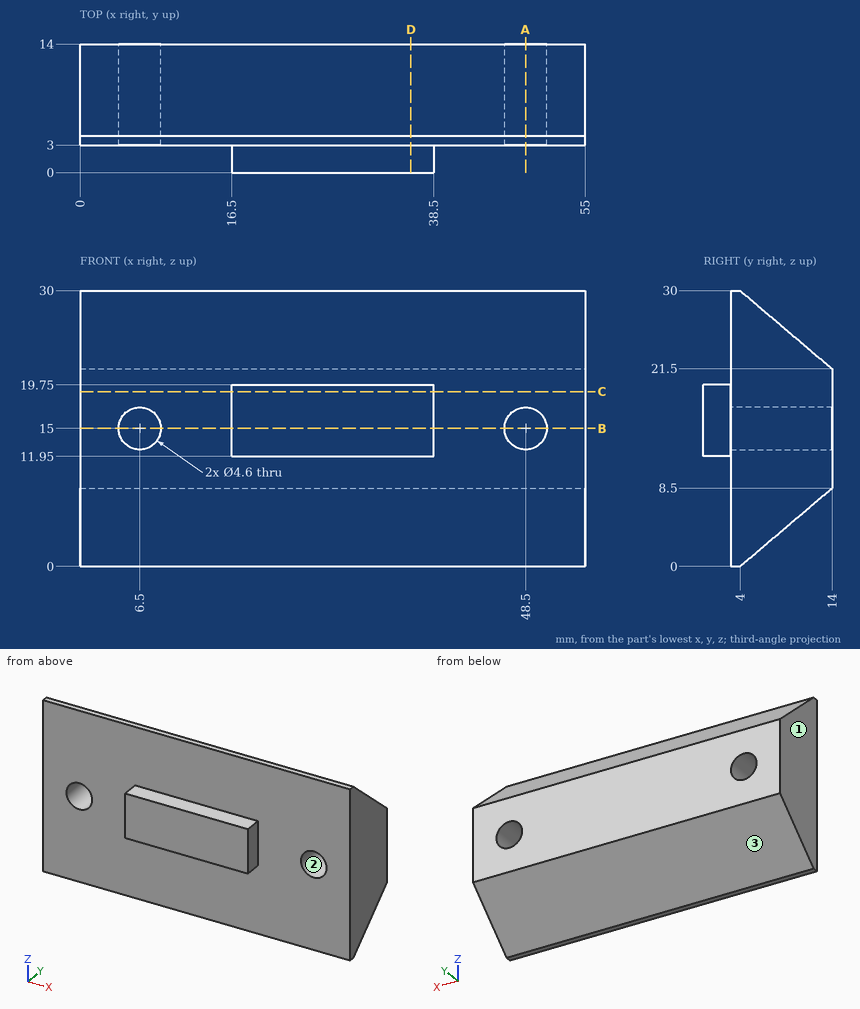
Input: dimensioned drawing with shaded views. Units: mm. Origin: part minimum x, y, z. Round coordinates to 2 decimals unless told otherwise and drop trailing zeros. Loops run counter-clockwise (first coordinate to the right, second up) from the corner with the lowest first, then second, coordinate; pieces in that order, holes last.
1) Section query A-A on x = 48.5. Return the cut outline in (y, z).
Ans:
outline: (3, 0) - (4, 0) - (14, 8.5) - (14, 12.7) - (3, 12.7) - close; (3, 17.3) - (14, 17.3) - (14, 21.5) - (4, 30) - (3, 30) - close
2) Section query B-B on z = 15. Return the cut outline in (x, y).
Ans:
outline: (0, 3) - (4.2, 3) - (4.2, 14) - (0, 14) - close; (8.8, 3) - (16.5, 3) - (16.5, 0) - (38.5, 0) - (38.5, 3) - (46.2, 3) - (46.2, 14) - (8.8, 14) - close; (50.8, 3) - (55, 3) - (55, 14) - (50.8, 14) - close
3) Pull-direction query (X, two-part tool) for the marked faces 1, 2 and 3; classes: released by +X, released by -X, zero draft, split by the parting line, or undercut.
Ans:
face 1: released by -X
face 2: undercut
face 3: zero draft
4) Section query D-D on x = 36. Return the cut outline in (y, z), plus the area to 3 significant figures.
Ans:
outline: (0, 11.95) - (3, 11.95) - (3, 0) - (4, 0) - (14, 8.5) - (14, 21.5) - (4, 30) - (3, 30) - (3, 19.75) - (0, 19.75) - close
area: 268 mm2
5) Material intervals for line 1 (X direction, y = 8.5, z = 15); line 2 (X direction, y = 7.75, z = 13); line 3 (Z direction, x = 19, y = 2), sorted ascending.
Ans:
line 1: x = 0 to 4.2, 8.8 to 46.2, 50.8 to 55
line 2: x = 0 to 5.36, 7.64 to 47.36, 49.64 to 55
line 3: z = 11.95 to 19.75
6) Pin query (flat end, axial travel): pin 1 (4 mm diameter, centred on x = 48.5, z = 15, fed in from +Y); pin 2 (1.5 mm diameter, centred on x = 8, y = 11, fed in from +Z); pin 3 (0.9 mm diameter, centred on y = 1.5, z = 14.5, fed in from +X). Return the tip coordinate at first contact, or that it passes through.
Ans:
pin 1: passes through
pin 2: stops at z = 24.69
pin 3: stops at x = 38.5
7) Section query C-C on z = 19. Return the cut outline in (x, y), plus the area to 3 significant figures.
Ans:
outline: (0, 3) - (16.5, 3) - (16.5, 0) - (38.5, 0) - (38.5, 3) - (55, 3) - (55, 14) - (0, 14) - close
area: 671 mm2
